Design review of the part built by this model. Coordinates are the model's own, in mm. Face numbers are marked on the shaded views. A direction names the side the tool comes from. Round coordinates to 2 decimals unless told otherwise and drop trailing zeros. Write each loop counter-clockwise with the first axis right and the second up, starting at its lowest first coordinate (ties: lowest second). Pieces come first, ordered by that corner, then holes.
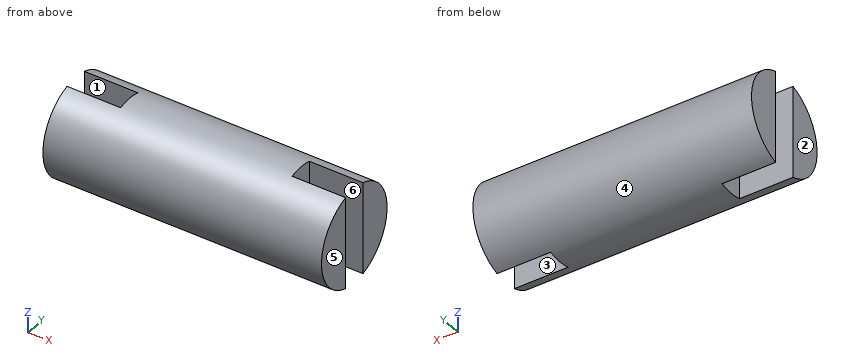
from build123d import *

# Parameters (mm, degrees)
F0_W     = 13
F0_H     = 2.25
F3_DEPTH = 2.5


# Not quite as in the source:
# - a pattern or mirror of a feature is missing from the dataset's text; its kind, count and spacing are read off the source's solid


with BuildPart() as f1:
    # F0 (on Front) → F1 (revolve)
    with BuildSketch(Plane.XZ):
        with Locations((6.5, 1.125)):
            Rectangle(F0_W, F0_H)
    revolve(axis=Axis((6.5, 0, 0), (1, 0, 0)))

    # F2 (on face) → F3 (cut)
    with BuildSketch(Plane.YZ.offset(13)):
        with BuildLine():
            Line((0.5940446135, -2.170163818), (0.5940446135, 2.170163818))
            ThreePointArc((0.5940446135, 2.170163818), (0, 2.25), (-0.5940446135, 2.170163818))
            Line((-0.5940446135, 2.170163818), (-0.5940446135, -2.170163818))
            ThreePointArc((-0.5940446135, -2.170163818), (0, -2.25), (0.5940446135, -2.170163818))
        make_face()
    f3 = extrude(amount=-F3_DEPTH, mode=Mode.SUBTRACT)

    # F3_copies: F3 across plane
    add(f3.mirror(Plane(origin=(6.5, 0, 0), x_dir=(0, 0, -1), z_dir=(-1, 0, 0))), mode=Mode.SUBTRACT)


solid = f1.part
1) The part is to be moulded in two halves that separate along Y. For the marked faces 3, 4, 5 and 6, say which applies: pulls with the +Y half, pulls with the -Y half, needs draft (parallel to the pull), parting line crosses it, or undercut.
2) Add section D-D on x = 3. State the section outline as (y, z) points.
3) For the marked faces 1 and 2, list the 3-axis set-ups (+Z, -Z, +X, -X, +Y, -Y) from which the entire face can be reached by the end or side of a thin tool; tool diameter is ignored.
4) For P1, Ø1, axis at x = 2.5, y = 1.5, coming from the +Z side; P2, Ø0.8, axis at x = 12.5, z = -1, coming from the -Y side; P3, Ø1, axis at y = 0, z = 0.5, coming from the -X side, all flat-tipped, find the tip position at first contact; note any pin that passes through.
5) For line 1 along X through (y, z) = (-0.4, 1.2); line 2 along Y through (x, z) = (12, 1.15); line 3 along Y through (x, z) = (4.25, -0.6), list the stretches that pass through material, from the lowest coordinate up.
6) Add section C-C on y = 0. State the section outline as (x, z) points, and give its area (3 significant figures).
7) Add section A-A on z = 0. State the section outline as (x, y) points.
8) Add section B-B on x = 11. State the section outline as (y, z) points, and give its area (3 significant figures).
Computed:
1. face 3: undercut
1. face 4: parting line crosses it
1. face 5: needs draft
1. face 6: undercut
2. outline: circle Ø4.5 at (0, 0)
3. face 1: +Z, -Z, -X
3. face 2: +Z, -Z, -X, +Y, -Y
4. P1: stops at z = 2.02
4. P2: stops at y = -2.17
4. P3: stops at x = 2.5
5. line 1: x = 2.5 to 10.5
5. line 2: y = -1.93 to -0.59, 0.59 to 1.93
5. line 3: y = -2.17 to 2.17
6. outline: (2.5, -2.25) - (10.5, -2.25) - (10.5, 2.25) - (2.5, 2.25) - close
6. area: 36.0 mm2
7. outline: (0, -2.25) - (13, -2.25) - (13, -0.59) - (10.5, -0.59) - (10.5, 0.59) - (13, 0.59) - (13, 2.25) - (0, 2.25) - (0, 0.59) - (2.5, 0.59) - (2.5, -0.59) - (0, -0.59) - close
8. outline: (-0.59, -2.17) - (-0.59, 2.17) arc R2.25 ccw to start; (0.59, -2.17) arc R2.25 ccw to (0.59, 2.17) - close
8. area: 10.6 mm2
